```python
from build123d import *

# Parameters (mm, degrees)
SKETCH010_R     = 1.75
PAD005_DEPTH    = 6.5
PAD006_DEPTH    = 10
SKETCH012_R     = 3
POCKET004_DEPTH = 14.45
SKETCH013_W     = 42.25
SKETCH013_H     = 43.25
SKETCH013_R     = 19.5
SKETCH013_R_2   = 1
PAD007_DEPTH    = 5
SKETCH054_W     = 13.95
SKETCH054_H     = 1
POCKET023_DEPTH = 1


with BuildPart() as part:
    # Sketch010 → Pad005 (new body)
    with BuildSketch(Plane.XZ):
        Polygon((14.45, 10), (14.45, -10), (-14.45, -10), (-14.45, 10), (-21.125, 31), (-21.125, 36), (21.125, 36), (21.125, 31), align=None)
        with Locations((-5, 7.5)):
            Circle(SKETCH010_R, mode=Mode.SUBTRACT)
        with Locations((5, 7.5)):
            Circle(SKETCH010_R, mode=Mode.SUBTRACT)
        with Locations((-5, -7.5)):
            Circle(SKETCH010_R, mode=Mode.SUBTRACT)
        with Locations((5, -7.5)):
            Circle(SKETCH010_R, mode=Mode.SUBTRACT)
    extrude(amount=PAD005_DEPTH)

    # Sketch011 → Pad006 (join)
    with BuildSketch(Plane.XZ):
        Polygon((-21.125, 36), (21.125, 36), (21.125, 31), (14.45, 10), (-14.45, 10), (-21.125, 31), align=None)
    extrude(amount=-PAD006_DEPTH)

    # Sketch012 → Pocket004 (cut, symmetric)
    with BuildSketch(Plane.YZ):
        with Locations((5, -14.5)):
            Circle(SKETCH012_R)
    extrude(amount=POCKET004_DEPTH, both=True, mode=Mode.SUBTRACT)

    # Sketch013 → Pad007 (join)
    with BuildSketch(Plane.XY.offset(36)):
        with Locations((0, 31.625)):
            Rectangle(SKETCH013_W, SKETCH013_H)
        with Locations((0, 30.240935)):
            Circle(SKETCH013_R, mode=Mode.SUBTRACT)
        with Locations((-16.25, 46.490935)):
            Circle(SKETCH013_R_2, mode=Mode.SUBTRACT)
        with Locations((16.25, 46.490935)):
            Circle(SKETCH013_R_2, mode=Mode.SUBTRACT)
        with Locations((16.25, 13.990935)):
            Circle(SKETCH013_R_2, mode=Mode.SUBTRACT)
        with Locations((-16.25, 13.990935)):
            Circle(SKETCH013_R_2, mode=Mode.SUBTRACT)
    extrude(amount=-PAD007_DEPTH)

    # Sketch054 → Pocket023 (cut)
    with BuildSketch(Plane.XZ):
        with Locations((-7.475, 0)):
            Rectangle(SKETCH054_W, SKETCH054_H)
        with Locations((7.475, 0)):
            Rectangle(SKETCH054_W, SKETCH054_H)
    extrude(amount=POCKET023_DEPTH, mode=Mode.SUBTRACT)


with BuildPart() as part_1:
    # Body003 placement: moved
    add(part.part.moved(Location((-30.55, -3.5, 0))))


solid = part_1.part
```
The listing builds one solid part. Answer for the finished solid, in the listing's coordinates (mm). A direction names the side the tool comes from. Give positions to 0.01 mm unless a question says otherwise; leave off trailing zeros. Loops run counter-clockwise (first coordinate to the right, second up) from the corner with the lowest first, then second, coordinate; pieces in that order, holes last. Notation, with made-up numbers: (35, 79) - (93, 79) arc R24 ccw to (93, 98) - close; hole circle Ø5 at (-35.75, -38.5). An arc over 180 degrees is marked (long way). Answer as CSV lines item,"result". Start each with the question number.
Item 1: The mould has two halves that part along X. Classify faces 3 (the face through (-15.3, 10.5, 33.5)), 4 (the face through (-47.8, 10.5, 33.5)), 5 (the face through (-9.425, 19, 34)), 6 (the face through (-45, -7, 0)): +X half, -X half, draft (parallel to the pull), parting line (faces both ways), or undercut.
Item 2: A cutting plane is placed at D-D on x = -14. Determine the outline of the cut face in (y, z), then the cut area to 3 significant figures.
Item 3: A cutting plane is placed at B-B on x = -43. Determine the outline of the cut face in (y, z), then the cut area to 3 significant figures.
Item 4: Each of these flat-tipped pins is pushed along its axis until it touches: pin 1 (5 mm diameter, centred on y = -6, z = 4.5, fed in from +X); pin 2 (12 mm diameter, centred on x = -14.5, y = 32, fed in from -Z); pin 3 (6 mm diameter, centred on x = -46.5, z = -5, fed in from +Y). Where does it stop, or does it pass through?
Item 5: A cutting plane is placed at C-C on y = 24.5. Determine the outline of the cut face in (x, z) (3 decimals), then the cut area to 3 significant figures.
Item 6: For faces 1 (the face through (-31, 7, 36)), 2 (the face through (-30.3, -3.5, 0.1)), determine the directions among +Z, -Z, +X, -X, +Y, -Y from which every point of the face is accessible in a straight line to the end or side of a thin tool.
Item 7: Find the intervals of material crossed by line 1 (Z direction, x = -25.55, y = -5.75); line 2 (Y direction, x = -30.55, z = 32.9); line 3 (Y direction, x = -14, z = 33), in increasing order. Write a range as from..to.
Item 8: A cutting plane is placed at A-A on z = -7.5. Determine the outline of the cut face in (x, y).
Found:
1,face 3,"undercut"
1,face 4,"undercut"
1,face 5,"+X half"
1,face 6,"-X half"
2,outline,"(-10, 16.61) - (6.5, 16.61) - (6.5, 31) - (9.54, 31) - (9.54, 36) - (-10, 36) - close; (11.44, 31) - (16.43, 31) - (16.43, 36) - (11.44, 36) - close; (37.05, 31) - (42.04, 31) - (42.04, 36) - (37.05, 36) - close; (43.94, 31) - (49.75, 31) - (49.75, 36) - (43.94, 36) - close"
2,area,"414 mm^2"
3,outline,"(-10, -10) - (-3.5, -10) - (-3.5, -0.5) - (-4.5, -0.5) - (-4.5, 0.5) - (-3.5, 0.5) - (-3.5, 10) - (6.5, 10) - (6.5, 31) - (11.73, 31) - (11.73, 36) - (-10, 36) - close; (41.75, 31) - (49.75, 31) - (49.75, 36) - (41.75, 36) - close"
3,area,"624 mm^2"
4,pin 1,"stops at x = -16.1"
4,pin 2,"stops at z = 31"
4,pin 3,"stops at y = -3.5"
5,outline,"(-51.675, 31) - (-49.921, 31) - (-49.921, 36) - (-51.675, 36) - close; (-11.179, 31) - (-9.425, 31) - (-9.425, 36) - (-11.179, 36) - close"
5,area,"17.5 mm^2"
6,face 1,"+Z, +X, -X, +Y, -Y"
6,face 2,"-Z, +X, -X, +Y"
7,line 1,"z = -10..-9.25, -5.75..5.75, 9.25..36"
7,line 2,"y = -10..7.24, 46.24..49.75"
7,line 3,"y = -10..9.54, 11.44..16.43, 37.05..42.04, 43.94..49.75"
8,outline,"(-45, -10) - (-37.3, -10) - (-37.3, -3.5) - (-45, -3.5) - close; (-33.8, -10) - (-27.3, -10) - (-27.3, -3.5) - (-33.8, -3.5) - close; (-23.8, -10) - (-16.1, -10) - (-16.1, -3.5) - (-23.8, -3.5) - close"
